Geometry check sheet. Reference: drawing and pictorial views, mm from the part's lowest x, y, z. A direction names the side the tool comes from. Give positions to 0.01 mm unless a question says otherwise; leave off trailing zeros. Order: outer loops, then holes, each group sorted by start corner. A loop starts at its lowest first (then second) coordinate and runs counter-clockwise, first axis right, second up. Notation, with made-up numbers: M 7.5,-30 L 51.5,-30 A15 ccw 51.5,-21 Z; hole C 81.25,89.25 d11. An arc over 180 degrees is marked long. Answer as CSV lines item,"result".
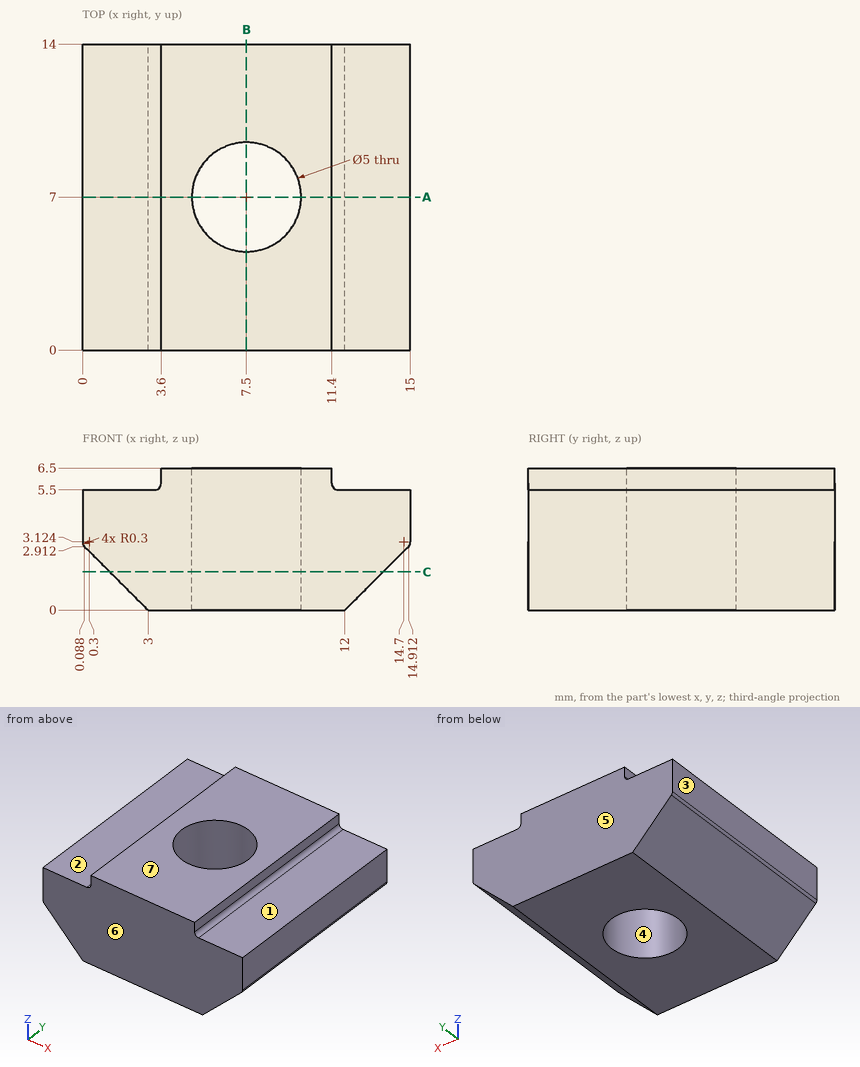
(1) Section check C-C on z = 1.75. Enter the section's corners in (x, y), then the cut area to 3 significant figures.
The answers:
outline,"M 1.25,0 L 13.75,0 L 13.75,14 L 1.25,14 Z; hole C 7.5,7 d5"
area,"155 mm2"
(2) Section check A-A on y = 7. Enter the section's corners in (x, z).
The answers:
outline,"M 0,3.12 A0.3 ccw 0.09,2.91 L 3,0 L 5,0 L 5,6.5 L 3.6,6.5 L 3.6,5.8 A0.3 cw 3.3,5.5 L 0,5.5 Z; M 10,0 L 12,0 L 14.91,2.91 A0.3 ccw 15,3.12 L 15,5.5 L 11.7,5.5 A0.3 cw 11.4,5.8 L 11.4,6.5 L 10,6.5 Z"
(3) Draft check along Y on the marked faces 4, 5, 6 and 7. Enter one of: +Y half, -Y half, draft (parallel to the pull), parting line (faces both ways), or undercut.
The answers:
face 4,"undercut"
face 5,"+Y half"
face 6,"-Y half"
face 7,"draft"
(4) Tool access check on the marked faces 1, 2 and 3. Record the directions out of +Z, -Z, +X, -X, +Y, -Y that give a thin tool (end or side, any length) a straight path to the whole face; none if there is none.
The answers:
face 1,"+Z, +X, +Y, -Y"
face 2,"+Z, -X, +Y, -Y"
face 3,"+Z, -Z, -X, +Y, -Y"
(5) Material ranges on line 1 (Y direction, x = 7.5, z = 3.5); line 2 (X direction, y = 7, z = 4.5); line 3 (Y direction, x = 7, z = 4.5), recorded low to high.
The answers:
line 1,"y = 0 to 4.5, 9.5 to 14"
line 2,"x = 0 to 5, 10 to 15"
line 3,"y = 0 to 4.55, 9.45 to 14"
(6) Gauge pin test, flat ends, axial feed: P1, Ø3.5, axis at x = 13.5, y = 7, coming from the +Z side; P2, Ø3, axis at x = 7.5, y = 7, coming from the +Z side. Record the tip position at first contact, or that the pin passes through.
The answers:
P1,"stops at z = 5.5"
P2,"passes through"
(7) Section check B-B on x = 7.5. Enter the section's corners in (y, z), then the cut area to 3 significant figures.
The answers:
outline,"M 0,0 L 4.5,0 L 4.5,6.5 L 0,6.5 Z; M 9.5,0 L 14,0 L 14,6.5 L 9.5,6.5 Z"
area,"58.5 mm2"
